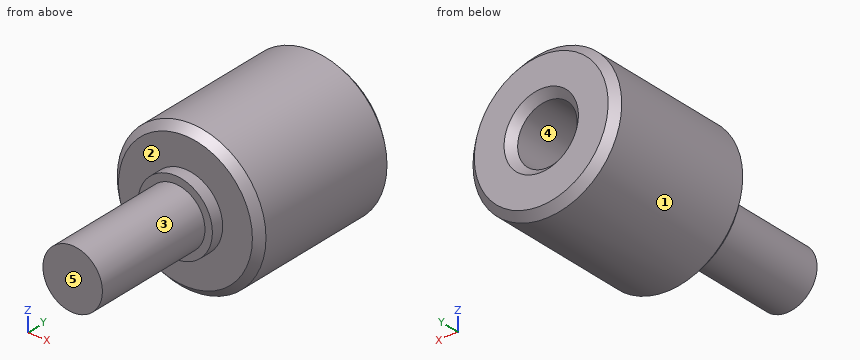
Autodesk Inventor part; units mm, degrees
ref_plane "YZ Plane" through (0, 0, 0) normal (1, 0, 0) x (0, 1, 0)
ref_plane "XZ Plane" through (0, 0, 0) normal (0, 1, 0) x (-1, 0, 0)
ref_plane "XY Plane" through (0, 0, 0) normal (0, 0, 1) x (1, 0, 0)
sketch "スケッチ1" plane through (0, 0, 0) normal (0, 0, 1) x (1, 0, 0)
  line L0 (0, -4.25) -> (0.9, -4.25)
  line L1 (0.9, -4.25) -> (1.2, -3.95)
  line L2 (1.2, -3.95) -> (1.2, 1.25)
  line L3 (1.2, 1.25) -> (1.5, 1.25)
  line L4 (1.5, 1.25) -> (1.5, 1.75)
  line L5 (1.5, 1.75) -> (2.7, 1.75)
  line L6 (3, 7.95) -> (2.7, 8.25)
  line L7 (2.7, 8.25) -> (1.5, 8.25)
  line L8 (1.5, 8.25) -> (1.2, 7.95)
  line L9 (0, 7.4044) -> (0, -7.4044) construction
  line L10 (0, -4.25) -> (0, 4.25)
  line L11 (0, 4.25) -> (1.2, 4.25)
  line L12 (1.2, 4.25) -> (1.2, 7.95)
  line L13 (2.7, 1.75) -> (3, 2.05)
  line L14 (3, 2.05) -> (3, 7.95)
  point P0 (0, 0)
  point P1 (0, 0)
  dimension "d0" = 2.4
  dimension "d1" = 6
  dimension "d2" = 0.3
  dimension "d3" = 0.3
  dimension "d4" = 3
  dimension "d5" = 0.5
  dimension "d6" = 6.5
  dimension "d8" = 0.3
  dimension "d9" = 2.4
  dimension "d10" = 4
  dimension "d11" = 0.3
  dimension "d12" = 0.3
  dimension "d13" = 0.3
  dimension "d14" = 0.3
  dimension "d15" = 6
revolve "回転1" add sketch "スケッチ1" angle 360 about axis through (0, 7.4044, 0) along (0, -1, 0)
sketch "スケッチ2" plane through (0, -4.25, 0) normal (0, -1, 0) x (1, 0, 0)
  circle A0 centre (0, 0) radius 0.9
  circle A1 centre (0, 0) radius 9.0242
extrude "押し出し1" cut sketch "スケッチ2" against normal blind 0.5 contours A0 | A1
equation "\"d3\" = d2"
equation "\"d11\" = d8"
equation "\"d12\" = d8"
equation "\"d13\" = d12"
equation "\"d14\" = d13"
properties part number "BRU-306_5" material "ステンレス鋼 AISI 304"
Work out the finished part from the listing and answer in its coordinate system (mm). Face numbers are marked on the shaded views. A direction names the side the tool comes from. Coordinates: 2 decimals unless noted, no trailing zeros. Loops run counter-clockwise (first coordinate to the right, second up) from the corner with the lowest first, then second, coordinate; pieces in that order, holes last. Notation, with made-up numbers: (-9, 46.25) -> (-4, 46.25) arc R16 ccw to (-4, 67.25) -> close; hole circle Ø6 at (63, 25.25). An arc over 180 degrees is marked (long way). Answer as CSV lines item,"result".
1) The part is cut by section B-B (y = 6.5). Give the vertices of the cut face in (x, z).
A:
outline,"circle Ø6 at (0, 0); hole circle Ø2.4 at (0, 0)"
2) The part is cut by section C-C (z = 0). Give the vertices of the cut face in (x, y).
A:
outline,"(-3, 2.05) -> (-2.7, 1.75) -> (-1.5, 1.75) -> (-1.5, 1.25) -> (-1.2, 1.25) -> (-1.2, -3.75) -> (1.2, -3.75) -> (1.2, 1.25) -> (1.5, 1.25) -> (1.5, 1.75) -> (2.7, 1.75) -> (3, 2.05) -> (3, 7.95) -> (2.7, 8.25) -> (1.5, 8.25) -> (1.2, 7.95) -> (1.2, 4.25) -> (-1.2, 4.25) -> (-1.2, 7.95) -> (-1.5, 8.25) -> (-2.7, 8.25) -> (-3, 7.95) -> close"
3) For a pull along X with two mould halves and no side action, classify the marked faces 3, 4 and 5 as released by +X, released by -X, zero draft, split by the parting line, or undercut.
A:
face 3,"split by the parting line"
face 4,"undercut"
face 5,"zero draft"
4) The part is cut by section D-D (y = 0.5). Give the vertices of the cut face in (x, z), and give its area (3 significant figures).
A:
outline,"circle Ø2.4 at (0, 0)"
area,"4.52 mm²"
5) For the marked faces 1 and 2, determine the directions among +Z, -Z, +X, -X, +Y, -Y from which every point of the face is accessible in a straight line to the end or side of a thin tool.
A:
face 1,"+Y, -Y"
face 2,"-Y"
6) Flat-ended cylindrical pins translate along their axes: pin 1 (1 mm diameter, centred on x = -2, z = -1.5, fed in from -Y); pin 2 (2.5 mm diameter, centred on x = 0, z = 0, fed in from +Y); pin 3 (1.5 mm diameter, centred on x = 1, y = 6, fed in from +Z). Find the tip coordinate at first contact, or state that the pin passes through.
A:
pin 1,"stops at y = 1.75"
pin 2,"stops at y = 8"
pin 3,"stops at z = 2.99"
7) The part is cut by section A-A (x = 0). Give the vertices of the cut face in (y, z).
A:
outline,"(-3.75, -1.2) -> (1.25, -1.2) -> (1.25, -1.5) -> (1.75, -1.5) -> (1.75, -2.7) -> (2.05, -3) -> (7.95, -3) -> (8.25, -2.7) -> (8.25, -1.5) -> (7.95, -1.2) -> (4.25, -1.2) -> (4.25, 1.2) -> (7.95, 1.2) -> (8.25, 1.5) -> (8.25, 2.7) -> (7.95, 3) -> (2.05, 3) -> (1.75, 2.7) -> (1.75, 1.5) -> (1.25, 1.5) -> (1.25, 1.2) -> (-3.75, 1.2) -> close"
8) Straight lines are drawn through the part: probe 1 along Z at (x, y) = (0, 5.95); probe 2 along Y at (x, z) = (-2, 0.95); probe 3 along X at (y, z) = (6, -0.9). For each, find the intervals that lie inside material, in ascending order.
A:
probe 1,"z = -3 to -1.2, 1.2 to 3"
probe 2,"y = 1.75 to 8.25"
probe 3,"x = -2.86 to -0.79, 0.79 to 2.86"
